Geometry: final body of the model. Coordinates: model frame, mm. A direction names the side the tool comes from. Round coordinates to 2 decimals unless told otherwise and drop trailing zeros. Loops run counter-clockwise (first coordinate to the right, second up) from the corner with the lowest first, then second, coordinate; pieces in that order, holes last. Notation, with made-up numbers: M 22,44 L 49,44 A11 ccw 49,64 Z; hole C 28,47.5 d9. An arc over 180 degrees is marked long. Answer as a JSON object with one key per item and string values.
from build123d import *

# Parameters (mm, degrees)
F0_R     = 3.175
F1_DEPTH = 8.89
F2_R     = 1.8415
F3_DEPTH = 5.08
F0_R_2   = 5.08
F4_DEPTH = 2.54


with BuildPart() as f1:
    # F0 (on Top) → F1 (new body)
    with BuildSketch(Plane.XY):
        Circle(F0_R)
    extrude(amount=F1_DEPTH)

    # F2 (on face) → F3 (cut)
    with BuildSketch(Plane.XY.offset(8.89)):
        Circle(F2_R)
    extrude(amount=-F3_DEPTH, mode=Mode.SUBTRACT)

    # F0 (on Top) → F4 (join)
    with BuildSketch(Plane.XY):
        Circle(F0_R_2)
        Circle(F0_R, mode=Mode.SUBTRACT)
    extrude(amount=F4_DEPTH)


solid = f1.part
1) Reachability of faces 1 (the flat face through (0, 0, 0)), 2 (the cylindrical face through (-0.69, -3.1, 5.67)) from +Z, -Z, +X, -X, +Y, -Y: full face, straight path, thin tool, end or side. Return the list, or none.
Results:
{"face 1": "-Z, +X, -X, +Y, -Y", "face 2": "+Z"}
2) Section query A-A (y = 0). Return the cut outline in (x, z) (1 decimal), and give its area (3 significant figures).
Results:
{"outline": "M -5.1,0 L 5.1,0 L 5.1,2.5 L 3.2,2.5 L 3.2,8.9 L 1.8,8.9 L 1.8,3.8 L -1.8,3.8 L -1.8,8.9 L -3.2,8.9 L -3.2,2.5 L -5.1,2.5 Z", "area": "47.4 mm2"}
3) Ray query, line 1 (Y direction, x = 0, z = 7.45) (1 decimal); line 2 (Z direction, x = -0.25, y = 1.75); line 3 (Z direction, x = -0.5, y = -3.75). Return the intervals inside material, ascending.
Results:
{"line 1": "-3.2 to -1.8, 1.8 to 3.2", "line 2": "0 to 3.81", "line 3": "0 to 2.54"}
4) Section query D-D (z = 1.5). Return the cut outline in (x, y).
Results:
{"outline": "C 0,0 d10.16"}
5) Pull-direction query (Y, two-part tool) for faces 3 (the cylindrical face through (-0.661, 5.037, 1.252)), 4 (the flat face through (0, -2, 8.89)), 5 (the cylindrical face through (0.85, -1.634, 6.386)); classes: +Y half, -Y half, draft (parallel to the pull), parting line (faces both ways), or undercut.
Results:
{"face 3": "parting line", "face 4": "draft", "face 5": "undercut"}
6) Pin query (flat end, axial travel): P1, Ø5, axis at x = -1.5, z = 3.5, coming from the -Y side; P2, Ø1.5, axis at y = -3, z = 4.5, coming from the +X side; P3, Ø3, axis at x = 3.5, z = 7.5, coming from the -Y side; P4, Ø1.8, axis at x = -0.5, y = -0.5, coming from the +Z side. Return the tip coordinate at first contact, or that it passes through.
Results:
{"P1": "y = -5.08", "P2": "x = 2.24", "P3": "y = -2.47", "P4": "z = 3.81"}
